Here's how the part is built. I have some questions about the finished solid (model axes, mm). A direction names the side the tool comes from. Coordinates: 2 decimals unless noted, no trailing zeros. Write each loop counter-clockwise with the first axis right and the second up, starting at its lowest first coordinate (ties: lowest second). Pieces come first, ordered by that corner, then holes.
(1) Imagine slicing it at D-D, the plane y = 34. List the corners of the cut face in (x, z) for me.
(2) For pin 1 Ø10 at (x, z) = (-4.5, -19.5) entering from -Y; pin 2 Ø3.5 at (x, z) = (-6.5, 27) entering from +Y; pin 3 Ø3 at (x, z) = (0, -31) entering from -Y; pin 4 Ø0.5 at (x, y) = (3, 36.5) entering from -Z, each with a flat end and sliding along its axis, tell me the tip position at first contact or that it passes through.
(3) Which directions (+Z, -Z, +X, -X, +Y, -Y) give clear straight access to the entire face, cutting with the end or side of a thin tool? Please do faces 1 (the flat face through (0, 26, -28)), 2 (the flat face through (0, 0, 0)), 3 (the flat face through (0, 36, 20)).
(4) Imagine slicing it at C-C, the plane x = -13. List the corners of the cut face in (y, z) for me, plus the area to 3 significant figures.
(5) Imagine slicing it at A-A, the plane x = 0. List the corners of the cut face in (y, z) for me, plus the area to 3 significant figures.
(6) Imagine slicing it at B-B, the plane z = -31. List the corners of the cut face in (x, y) for me.
(7) Thinking about a two-plate mould opening in X: for faces 4 (the flat face through (16, 18, 0)), 5 (the cylindrical face through (-0.766, 12.818, 29.153)), 6 (the flat face through (0, 37, 0)), which applies, released by +X, released by -X, zero draft, split by the parting line, or undercut?
(8) Please list where these lines run through material, in increasing order: probe 1 along X at (y, z) = (7, -31); probe 2 along Z at (x, y) = (-0.5, 9); probe 3 along Y at (x, z) = (8, -27).
```python
from build123d import *

# Parameters (mm, degrees)
SKETCH_1_W          = 32
SKETCH_1_H          = 70
EXTRUDE_1_DEPTH     = 26
SKETCH_2_W          = 36
SKETCH_2_H          = 1
EXTRUDE_2_DEPTH     = 32
SKETCH_3_R          = 2
CUT_EXTRUDE_1_DEPTH = 54.38539126


with BuildPart() as part:
    # ｽｹｯﾁ1 → ﾎﾞｽ - 押し出し1 (new body)
    with BuildSketch(Plane(origin=(0, 0, 0), x_dir=(1, 0, 0), z_dir=(0, 1, 0))):
        Rectangle(SKETCH_1_W, SKETCH_1_H)
    extrude(amount=EXTRUDE_1_DEPTH)

    # ｽｹｯﾁ2 → ﾎﾞｽ - 押し出し2 (add)
    with BuildSketch(Plane(origin=(16, 0, 0), x_dir=(0, 0, -1), z_dir=(1, 0, 0))):
        Polygon((-18, 36), (-22, 36), (-22, 26), (22, 26), (22, 36), (18, 36), align=None)
        with Locations((0, 36.5)):
            Rectangle(SKETCH_2_W, SKETCH_2_H)
        Polygon((-22, 26), (-22, 36), (-23.75, 26), align=None)
        Polygon((22, 36), (22, 26), (23.75, 26), align=None)
    extrude(amount=-EXTRUDE_2_DEPTH)

    # ｽｹｯﾁ3 → ｶｯﾄ - 押し出し1 (cut, through all)
    with BuildSketch(Plane.XZ):
        with Locations(Location((0, 31, 0), (0, 0, 270))):
            Circle(SKETCH_3_R)
        with Locations(Location((0, -31, 0), (0, 0, 90))):
            Circle(SKETCH_3_R)
    extrude(amount=-CUT_EXTRUDE_1_DEPTH, mode=Mode.SUBTRACT)


solid = part.part
```
Recorded:
1. outline: (-16, -22.35) - (16, -22.35) - (16, 22.35) - (-16, 22.35) - close
2. pin 1: stops at y = 0
2. pin 2: stops at y = 26
2. pin 3: passes through
2. pin 4: stops at z = -18
3. face 1: -Z, +X, -X, +Y
3. face 2: +Z, -Z, +X, -X, -Y
3. face 3: +Z, +X, -X, +Y
4. outline: (0, -35) - (26, -35) - (26, -23.75) - (36, -22) - (36, -18) - (37, -18) - (37, 18) - (36, 18) - (36, 22) - (26, 23.75) - (26, 35) - (0, 35) - close
4. area: 2,310 mm2
5. outline: (0, -35) - (26, -35) - (26, -33) - (0, -33) - close; (0, -29) - (26, -29) - (26, -23.75) - (36, -22) - (36, -18) - (37, -18) - (37, 18) - (36, 18) - (36, 22) - (26, 23.75) - (26, 29) - (0, 29) - close; (0, 33) - (26, 33) - (26, 35) - (0, 35) - close
5. area: 2,110 mm2
6. outline: (-16, 0) - (-2, 0) - (-2, 26) - (-16, 26) - close; (2, 0) - (16, 0) - (16, 26) - (2, 26) - close
7. face 4: released by +X
7. face 5: undercut
7. face 6: zero draft
8. probe 1: x = -16 to -2, 2 to 16
8. probe 2: z = -35 to -32.94, -29.06 to 29.06, 32.94 to 35
8. probe 3: y = 0 to 26
